from build123d import *

# Parameters (mm, degrees)
BASE_FLANGE1_DEPTH    = 30
F_3_0MM_DOWEL_HOLE1_D = 3


# Sheet-metal steps are written as plain solids
with BuildPart() as part:
    # Sketch1 → Base-Flange1 (new body)
    with BuildSketch(Plane.XY):
        with BuildLine():
            Line((0, 0), (0, 17.7634))
            ThreePointArc((0, 17.7634), (0.655084973, 19.344915027), (2.2366, 20))
            Line((2.2366, 20), (10, 20))
            Line((10, 20), (10, 18.5))
            Line((10, 18.5), (2.2366, 18.5))
            ThreePointArc((2.2366, 18.5), (1.715745145, 18.284254855), (1.5, 17.7634))
            Line((1.5, 17.7634), (1.5, 0))
            Line((1.5, 0), (0, 0))
        make_face()
    extrude(amount=BASE_FLANGE1_DEPTH)

    # Ø3.0mm Dowel Hole1 (through all)
    with Locations(Plane(origin=(5.118724392, 18.5, 37.745569698), x_dir=(-1, 0, 0), z_dir=(0, -1, 0))):
        with Locations((-0.881275608, 12.745569698)):
            Hole(F_3_0MM_DOWEL_HOLE1_D / 2)


solid = part.part
Source: CAD feature listing. Evaluate the final solid. Frame: model axes, mm. A direction names the side the tool comes from. Coordinates: 2 decimals unless noted, no trailing zeros. Loops run counter-clockwise (first coordinate to the right, second up) from the corner with the lowest first, then second, coordinate; pieces in that order, holes last. Notation, with made-up numbers: (86, 72) - (104, 72) arc R19 ccw to (104, 104) - close; hole circle Ø1 at (-11.75, -34). An arc over 180 degrees is marked (long way). One line per item, written item: value. Start each with the question number.
1. Section D-D (y = 11.75). Return the cut outline in (x, z), and give its area (3 significant figures).
2. Set-up query: faces 4 (the flat face through (1, 0, 15)), 5 (the flat face through (6, 18.5, 15)). Return all of +Z, -Z, +X, -X, +Y, -Y with unobstructed straight access to the full face (end or side cutting, diameter ignored); none if empty.
3. Ray query, L1, parallel to Z at x = 6, y = 19.5; L2, parallel to X at y = 19.45, z = 25; L3, parallel to X at y = 16, z = 12. Return the intervals inside material, ascending.
4. Section B-B (x = 6). Return the cut outline in (y, z).
5. Mould query, pull axis Z, two halves, no side actions, for faces 1 (the flat face through (1.5, 9, 15)), 2 (the cylindrical face through (5.805, 19.26, 23.513)), 3 (the flat face through (1, 13, 0)). Classes: pulls with the +Z half, pulls with the -Z half, needs draft (parallel to the pull), parting line crosses it, or undercut.
6. Section C-C (z = 17). Return the cut outline in (x, y), and give its area (3 significant figures).
7. Section A-A (z = 25). Return the cut outline in (x, y).
8. Contact query for flat-ended pins moving along their axis: P1, Ø6, axis at x = 6, z = 12, coming from the -Y side; P2, Ø3, axis at x = 4, y = 10, coming from the -Z side; P3, Ø1.5, axis at y = 6.5, z = 16.5, coming from the +X side. Output: stop coordinate, or through.
Verdict:
1. outline: (0, 0) - (1.5, 0) - (1.5, 30) - (0, 30) - close
1. area: 45.0 mm2
2. face 4: +Z, -Z, +X, -X, -Y
2. face 5: +Z, -Z, +X, -Y
3. L1: z = 0 to 23.5, 26.5 to 30
3. L2: x = 0.77 to 4.5, 7.5 to 10
3. L3: x = 0 to 1.5
4. outline: (18.5, 0) - (20, 0) - (20, 23.5) - (18.5, 23.5) - close; (18.5, 26.5) - (20, 26.5) - (20, 30) - (18.5, 30) - close
5. face 1: needs draft
5. face 2: undercut
5. face 3: pulls with the -Z half
6. outline: (0, 0) - (1.5, 0) - (1.5, 17.76) arc R0.74 cw to (2.24, 18.5) - (10, 18.5) - (10, 20) - (2.24, 20) arc R2.24 ccw to (0, 17.76) - close
6. area: 41.8 mm2
7. outline: (0, 0) - (1.5, 0) - (1.5, 17.76) arc R0.74 cw to (2.24, 18.5) - (4.5, 18.5) - (4.5, 20) - (2.24, 20) arc R2.24 ccw to (0, 17.76) - close; (7.5, 18.5) - (10, 18.5) - (10, 20) - (7.5, 20) - close
8. P1: stops at y = 18.5
8. P2: passes through
8. P3: stops at x = 1.5
